Check sheet for the modelled part. Datum: model origin and axes. Units: mm. Face numbers are marked on the shaded views. A direction names the side the tool comes from. Round coordinates to 2 decimals unless told otherwise and drop trailing zeros. Write each loop counter-clockwise with the first axis right and the second up, starting at its lowest first coordinate (ties: lowest second). Pieces come first, ordered by that corner, then holes. Notation, with made-up numbers: (69.25, 44.5) -> (79.25, 44.5) arc R24 cw to (79.25, 82.5) -> close; hole circle Ø3 at (-0.5, -11). An arc over 180 degrees is marked (long way). Answer as a JSON object with one key per item and string values. Group by question number.
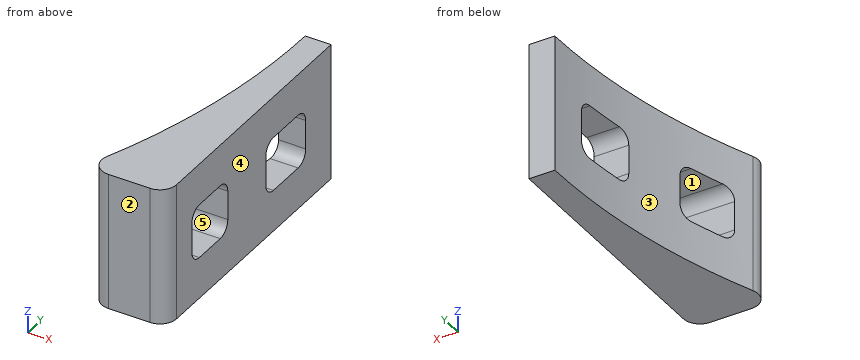
```python
from build123d import *

# Parameters (mm, degrees)
RESSALTO_EXTRUS_O1_DEPTH = 33
CORTE_EXTRUS_O1_DEPTH    = 33
FILETE1_R                = 4


with BuildPart() as part:
    # Esboço1 → Ressalto-extrusão1 (new body)
    with BuildSketch(Plane.XY):
        with BuildLine():
            Line((-20.29157915, 93.135393664), (-14.089663978, 93.135393664))
            Line((-14.089663978, 93.135393664), (-14.089663978, 28.135393664))
            Line((-14.089663978, 28.135393664), (-34.089663978, 28.135393664))
            ThreePointArc((-34.089663978, 28.135393664), (-23.779109315, 59.911203888), (-20.29157915, 93.135393664))
        make_face()
    extrude(amount=RESSALTO_EXTRUS_O1_DEPTH)

    # Esboço2 → Corte-extrusão1 (cut)
    with BuildSketch(Plane(origin=(-14.089663978, 0, 0), x_dir=(0, 0, -1), z_dir=(1, 0, 0))):
        with BuildLine():
            Line((-20, 83.135393664), (-13, 83.135393664))
            ThreePointArc((-13, 83.135393664), (-10.878679656, 82.256714007), (-10, 80.135393664))
            Line((-10, 80.135393664), (-10, 70.356838266))
            ThreePointArc((-10, 70.356838266), (-10.878679656, 68.235517922), (-13, 67.356838266))
            Line((-13, 67.356838266), (-20, 67.356838266))
            ThreePointArc((-20, 67.356838266), (-22.121320344, 68.235517922), (-23, 70.356838266))
            Line((-23, 70.356838266), (-23, 80.135393664))
            ThreePointArc((-23, 80.135393664), (-22.121320344, 82.256714007), (-20, 83.135393664))
        make_face()
        with BuildLine():
            Line((-20, 52.356838266), (-13, 52.356838266))
            ThreePointArc((-13, 52.356838266), (-10.878679656, 51.478158609), (-10, 49.356838266))
            Line((-10, 49.356838266), (-10, 41.135393664))
            ThreePointArc((-10, 41.135393664), (-10.878679656, 39.01407332), (-13, 38.135393664))
            Line((-13, 38.135393664), (-20, 38.135393664))
            ThreePointArc((-20, 38.135393664), (-22.121320344, 39.01407332), (-23, 41.135393664))
            Line((-23, 41.135393664), (-23, 49.356838266))
            ThreePointArc((-23, 49.356838266), (-22.121320344, 51.478158609), (-20, 52.356838266))
        make_face()
    extrude(amount=-CORTE_EXTRUS_O1_DEPTH, mode=Mode.SUBTRACT)

    # Filete1
    filete1_edges = [part.edges().sort_by_distance(p)[0] for p in [
        (-14.089663978, 28.135393664, 16.5),
        (-34.089663978, 28.135393664, 16.5),
    ]]
    fillet(filete1_edges, radius=FILETE1_R)


solid = part.part
```
(1) Scan lines: line 1 along Y through (x, z) = (-19, 18); line 2 along Y through (x, z) = (-16, 16.5); line 3 along Z through (x, y) = (-16, 74). Record each from-to range of solid material in increasing order.
(2) Section check D-D on x = -19.5. Record the cut outline in (y, z).
(3) Access from +Z, -Z, +X, -X, +Y, -Y to the whole of each face (thin tool, end or side, straight path). Record for the marked faces 1 and 2.
(4) Section check C-C on x = -24.5. Record the cut outline in (y, z).
(5) Section check B-B on y = 74. Record the cut outline in (x, z).
(6) Go/stop test with flat-tipped pins: pin 1 Ø2 at (y, z) = (80, 29.5) entering from -X; pin 2 Ø8 at (y, z) = (52.5, 10) entering from -X; pin 3 Ø2 at (y, z) = (62, 23.5) entering from -X. Record where each tip stops, or that it passes through.
(7) Section check A-A on z = 14.5. Record the cut outline in (x, y).
(8) Release check for a two-part mould opening along Y. For the marked faces 3, 4 and 5 record: pulls with the +Y half, pulls with the -Y half, needs draft (parallel to the pull), parting line crosses it, or undercut.
Data:
{
 "1": {"line 1": "y = 28.14 to 38.14, 52.36 to 67.36, 83.14 to 93.14", "line 2": "y = 28.72 to 38.14, 52.36 to 67.36, 83.14 to 93.14", "line 3": "z = 0 to 10, 23 to 33"},
 "2": {"outline": "(28.14, 0) -> (93.14, 0) -> (93.14, 33) -> (28.14, 33) -> close; hole (38.14, 13) arc R3 ccw to (41.14, 10) -> (49.36, 10) arc R3 ccw to (52.36, 13) -> (52.36, 20) arc R3 ccw to (49.36, 23) -> (41.14, 23) arc R3 ccw to (38.14, 20) -> close; hole (67.36, 13) arc R3 ccw to (70.36, 10) -> (80.14, 10) arc R3 ccw to (83.14, 13) -> (83.14, 20) arc R3 ccw to (80.14, 23) -> (70.36, 23) arc R3 ccw to (67.36, 20) -> close"},
 "3": {"face 1": "+X, -X", "face 2": "+Z, -Z, +X, -X, -Y"},
 "4": {"outline": "(28.14, 0) -> (56.68, 0) -> (56.68, 33) -> (28.14, 33) -> close; hole (38.14, 13) arc R3 ccw to (41.14, 10) -> (49.36, 10) arc R3 ccw to (52.36, 13) -> (52.36, 20) arc R3 ccw to (49.36, 23) -> (41.14, 23) arc R3 ccw to (38.14, 20) -> close"},
 "5": {"outline": "(-21.44, 0) -> (-14.09, 0) -> (-14.09, 10) -> (-21.44, 10) -> close; (-21.44, 23) -> (-14.09, 23) -> (-14.09, 33) -> (-21.44, 33) -> close"},
 "6": {"pin 1": "stops at x = -20.92", "pin 2": "stops at x = -26.64", "pin 3": "stops at x = -23.55"},
 "7": {"outline": "(-31.77, 33.62) arc R4 ccw to (-28.06, 28.14) -> (-18.09, 28.14) arc R4 ccw to (-14.09, 32.14) -> (-14.09, 38.14) -> (-30.04, 38.14) arc R160 cw to start; (-25.58, 52.36) -> (-14.09, 52.36) -> (-14.09, 67.36) -> (-22.38, 67.36) arc R160 cw to start; (-20.6, 83.14) -> (-14.09, 83.14) -> (-14.09, 93.14) -> (-20.29, 93.14) arc R160 cw to start"},
 "8": {"face 3": "pulls with the +Y half", "face 4": "needs draft", "face 5": "undercut"}
}
